from build123d import *

# Parameters (mm, degrees)
F0_W     = 76.2
F0_H     = 50.8
F0_R     = 12.7
F1_DEPTH = 12.7
F2_W     = 1.27
F2_H     = 50.8
F3_DEPTH = 5.08
F5_DEPTH = 50.801
F6_R     = 4.445
F7_DEPTH = 12.7


with BuildPart() as f1:
    # F0 (on Top) → F1 (new body)
    with BuildSketch(Plane.XY):
        Rectangle(F0_W, F0_H)
        Circle(F0_R, mode=Mode.SUBTRACT)
    extrude(amount=F1_DEPTH)

    # F2 (on face) → F3 (cut)
    with BuildSketch(Plane.XY.offset(12.7)):
        with Locations((-27.305, 0)):
            Rectangle(F2_W, F2_H)
        with BuildLine():
            Line((6.35, 25.4), (-6.35, 25.4))
            Line((-6.35, 25.4), (-6.35, 10.9985226281))
            ThreePointArc((-6.35, 10.9985226281), (0, 12.7), (6.35, 10.9985226281))
            Line((6.35, 10.9985226281), (6.35, 25.4))
        make_face()
        with BuildLine():
            Line((-6.35, -10.9985226281), (-6.35, -25.4))
            Line((-6.35, -25.4), (6.35, -25.4))
            Line((6.35, -25.4), (6.35, -10.9985226281))
            ThreePointArc((6.35, -10.9985226281), (0, -12.7), (-6.35, -10.9985226281))
        make_face()
    extrude(amount=-F3_DEPTH, mode=Mode.SUBTRACT)

    # F4 (on face) → F5 (cut, through all)
    with BuildSketch(Plane.XZ.offset(25.4)):
        Polygon((25.4, 12.7), (19.05, 12.7), (16.1170606325, 7.62), (25.4, 7.62), align=None)
        Polygon((31.75, 12.7), (25.4, 12.7), (25.4, 7.62), (34.6829393675, 7.62), align=None)
    extrude(amount=-F5_DEPTH, mode=Mode.SUBTRACT)

    # F6 (on face) → F7 (join)
    with BuildSketch(Plane.YZ.offset(38.1)):
        with Locations((0, 6.35)):
            Circle(F6_R)
    extrude(amount=F7_DEPTH)


solid = f1.part
Source: CAD feature listing. Evaluate the final solid. Frame: model axes, mm. A direction names the side the tool comes from. Coordinates: 2 decimals unless noted, no trailing zeros. Loops run counter-clockwise (first coordinate to the right, second up) from the corner with the lowest first, then second, coordinate; pieces in that order, holes last. Notation, with made-up numbers: (56.25, 16) -> (107.25, 16) arc R37 cw to (107.25, 54) -> close; hole circle Ø4 at (-33, 39). An arc over 180 degrees is marked (long way). Answer in a Markdown table with one row per item. Add a question column.
Q1. Reachability of faces 4 (the face through (-26.67, 0, 10)), 5 (the face through (25, 0, 7.62)), 6 (the face through (-33, 0, 12.7)) from +Z, -Z, +X, -X, +Y, -Y: full face, straight path, thin tool, end or side. Return the list, or none.
Q2. Section B-B on x = 0. Return the cut outline in (y, z), and give its area (3 significant figures).
Q3. Section C-C on z = 6.35. Return the cut outline in (x, y) (3 decimals), and give its area (3 significant figures).
Q4. Pull-direction query (Z, two-part tool) for faces 1 (the face through (33.24, -0.36, 10.12)), 2 (the face through (-17, 0, 12.7)), 3 (the face through (-1.653, 12.592, 6.261)); classes: pulls with the +Z half, pulls with the -Z half, needs draft (parallel to the pull), parting line crosses it, or undercut.
Q5. Section A-A on y = 0. Return the cut outline in (x, z) (3 decimals).
Q6. Ray query, line 1 along X through (y, z) = (0, 3.75); line 2 along X through (y, z) = (11, 7); line 3 along X through (y, z) = (0, 8.5). Return the intervals inside material, ascending.
Q7. Section D-D on y = -20. Return the cut outline in (x, z).
Q8. Contact query for flat-ended pins moving along their axis: pin 1 Ø10 at (x, y) = (0, 16) entering from +Z; pin 2 Ø6 at (y, z) = (-12, 10) entering from +X. Output: stop coordinate, or through.
Computed values:
| question | item | result |
|---|---|---|
| 1 | face 4 | +Z, +Y, -Y |
| 1 | face 5 | +Y, -Y |
| 1 | face 6 | +Z, +X, -X, +Y, -Y |
| 2 | outline | (-25.4, 0) -> (-12.7, 0) -> (-12.7, 7.62) -> (-25.4, 7.62) -> close; (12.7, 0) -> (25.4, 0) -> (25.4, 7.62) -> (12.7, 7.62) -> close |
| 2 | area | 194 mm^2 |
| 3 | outline | (-38.1, -25.4) -> (38.1, -25.4) -> (38.1, -4.445) -> (50.8, -4.445) -> (50.8, 4.445) -> (38.1, 4.445) -> (38.1, 25.4) -> (-38.1, 25.4) -> close; hole circle Ø25.4 at (0, 0) |
| 3 | area | 3,480 mm^2 |
| 4 | face 1 | undercut |
| 4 | face 2 | pulls with the +Z half |
| 4 | face 3 | needs draft |
| 5 | outline | (-38.1, 0) -> (-12.7, 0) -> (-12.7, 12.7) -> (-26.67, 12.7) -> (-26.67, 7.62) -> (-27.94, 7.62) -> (-27.94, 12.7) -> (-38.1, 12.7) -> close; (12.7, 0) -> (38.1, 0) -> (38.1, 1.905) -> (50.8, 1.905) -> (50.8, 10.795) -> (38.1, 10.795) -> (38.1, 12.7) -> (31.75, 12.7) -> (34.683, 7.62) -> (16.117, 7.62) -> (19.05, 12.7) -> (12.7, 12.7) -> close |
| 6 | line 1 | x = -38.1 to -12.7, 12.7 to 50.8 |
| 6 | line 2 | x = -38.1 to -6.35, 6.35 to 38.1 |
| 6 | line 3 | x = -38.1 to -27.94, -26.67 to -12.7, 12.7 to 16.63, 34.17 to 50.8 |
| 7 | outline | (-38.1, 0) -> (38.1, 0) -> (38.1, 12.7) -> (31.75, 12.7) -> (34.68, 7.62) -> (16.12, 7.62) -> (19.05, 12.7) -> (6.35, 12.7) -> (6.35, 7.62) -> (-6.35, 7.62) -> (-6.35, 12.7) -> (-26.67, 12.7) -> (-26.67, 7.62) -> (-27.94, 7.62) -> (-27.94, 12.7) -> (-38.1, 12.7) -> close |
| 8 | pin 1 | stops at z = 7.62 |
| 8 | pin 2 | stops at x = 38.1 |
